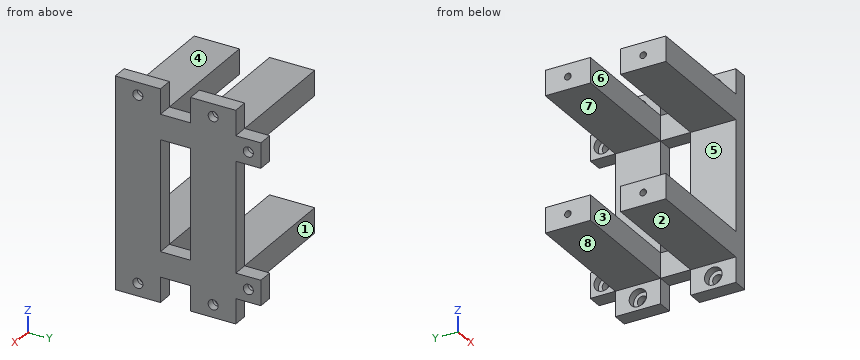
```python
from build123d import *

# Parameters (mm, degrees)
SKETCH_1_W           = 32
SKETCH_1_H           = 24
EXTRUDE_1_DEPTH      = 23.8
SKETCH_7_R           = 0.65
CUT_EXTRUDE_1_DEPTH  = 2
SKETCH_8_OUTSIDE_W   = 43.31
SKETCH_8_OUTSIDE_H   = 35.31
SKETCH_8_OUTSIDE_W_2 = 5
SKETCH_8_OUTSIDE_H_2 = 9
CUT_EXTRUDE_2_DEPTH  = 32.087618114
SKETCH_9_R           = 1
SKETCH_9_W           = 22
SKETCH_9_H           = 6
EXTRUDE_2_DEPTH      = 3
SKETCH_11_R          = 1.75
CUT_EXTRUDE_3_DEPTH  = 1.5


with BuildPart() as part:
    # Sketch 1 → Extrude 1 (new body)
    with BuildSketch(Plane(origin=(0, 0, 0), x_dir=(0, 0, -1), z_dir=(1, 0, 0))):
        Rectangle(SKETCH_1_W, SKETCH_1_H)
    extrude(amount=EXTRUDE_1_DEPTH)

    # Sketch 7 → Cut-Extrude 1 (cut)
    with BuildSketch(Plane.ZY):
        with Locations((13.5, 7.5)):
            Circle(SKETCH_7_R)
        with Locations((13.5, -7.5)):
            Circle(SKETCH_7_R)
        with Locations((-13.5, -7.5)):
            Circle(SKETCH_7_R)
        with Locations((-13.5, 7.5)):
            Circle(SKETCH_7_R)
    extrude(amount=-CUT_EXTRUDE_1_DEPTH, mode=Mode.SUBTRACT)

    # Sketch 8 outside → Cut-Extrude 2 (cut, through all)
    with BuildSketch(Plane.ZY):
        Rectangle(SKETCH_8_OUTSIDE_W, SKETCH_8_OUTSIDE_H)
        with Locations((-13.5, -7.5)):
            Rectangle(SKETCH_8_OUTSIDE_W_2, SKETCH_8_OUTSIDE_H_2, mode=Mode.SUBTRACT)
        with Locations((-13.5, 7.5)):
            Rectangle(SKETCH_8_OUTSIDE_W_2, SKETCH_8_OUTSIDE_H_2, mode=Mode.SUBTRACT)
        with Locations((13.5, -7.5)):
            Rectangle(SKETCH_8_OUTSIDE_W_2, SKETCH_8_OUTSIDE_H_2, mode=Mode.SUBTRACT)
        with Locations((13.5, 7.5)):
            Rectangle(SKETCH_8_OUTSIDE_W_2, SKETCH_8_OUTSIDE_H_2, mode=Mode.SUBTRACT)
    extrude(amount=-CUT_EXTRUDE_2_DEPTH, mode=Mode.SUBTRACT)


with BuildPart() as cut_extrude_2_piece_1:
    # of the separate pieces the step leaves, piece 1, a body of its own (cut_extrude_2_pieces)
    add(part.part.solids().sort_by_distance((0, 12, 16))[0])



with BuildPart() as cut_extrude_2_piece_2:
    # of the separate pieces the step leaves, piece 2, a body of its own (cut_extrude_2_pieces)
    add(part.part.solids().sort_by_distance((0, -12, 16))[0])


with BuildPart() as cut_extrude_2_piece_3:
    # of the separate pieces the step leaves, piece 3, a body of its own (cut_extrude_2_pieces)
    add(part.part.solids().sort_by_distance((0, 3, -11))[0])


with BuildPart() as cut_extrude_2_piece_4:
    # of the separate pieces the step leaves, piece 4, a body of its own (cut_extrude_2_pieces)
    add(part.part.solids().sort_by_distance((0, -12, -11))[0])


with BuildPart() as cut_extrude_2_piece_1_1:
    add(cut_extrude_2_piece_1.part)

    add(cut_extrude_2_piece_2.part)  # Extrude 2 merges Cut-Extrude 2 piece 2

    add(cut_extrude_2_piece_3.part)  # Extrude 2 merges Cut-Extrude 2 piece 3

    add(cut_extrude_2_piece_4.part)  # Extrude 2 merges Cut-Extrude 2 piece 4
    # Sketch 9 → Extrude 2 (add)
    with BuildSketch(Plane(origin=(23.8, 0, 0), x_dir=(0, 0, -1), z_dir=(1, 0, 0))):
        Polygon((16, -3), (16, 3), (21, 3), (21, 12), (16, 12), (16, 17), (11, 17), (11, 12), (-11, 12), (-11, 17), (-16, 17), (-16, 12), (-21, 12), (-21, 3), (-16, 3), (-16, -3), (-21, -3), (-21, -12), (21, -12), (21, -3), align=None)
        with Locations((18.5, 7.5)):
            Circle(SKETCH_9_R, mode=Mode.SUBTRACT)
        with Locations((13.5, 14.5)):
            Circle(SKETCH_9_R, mode=Mode.SUBTRACT)
        with Locations((-18.5, -7.5)):
            Circle(SKETCH_9_R, mode=Mode.SUBTRACT)
        with Locations((18.5, -7.5)):
            Circle(SKETCH_9_R, mode=Mode.SUBTRACT)
        Rectangle(SKETCH_9_W, SKETCH_9_H, mode=Mode.SUBTRACT)
        with Locations((-18.5, 7.5)):
            Circle(SKETCH_9_R, mode=Mode.SUBTRACT)
        with Locations((-13.5, 14.5)):
            Circle(SKETCH_9_R, mode=Mode.SUBTRACT)
    extrude(amount=EXTRUDE_2_DEPTH)

    # Sketch 11 → Cut-Extrude 3 (cut)
    with BuildSketch(Plane.ZY.offset(-23.8)):
        with Locations((-18.5, -7.5)):
            Circle(SKETCH_11_R)
        with Locations((-13.5, -14.5)):
            Circle(SKETCH_11_R)
        with Locations((-18.546966213, 7.5)):
            Circle(SKETCH_11_R)
        with Locations((13.5, -14.5)):
            Circle(SKETCH_11_R)
        with Locations((18.5, -7.5)):
            Circle(SKETCH_11_R)
        with Locations((18.5, 7.5)):
            Circle(SKETCH_11_R)
        with Locations((13.5, 14.5)):
            Circle(SKETCH_11_R)
        with Locations((-13.5, 14.5)):
            Circle(SKETCH_11_R)
    extrude(amount=-CUT_EXTRUDE_3_DEPTH, mode=Mode.SUBTRACT)


solid = cut_extrude_2_piece_1_1.part
```
Could you check a few things on this model? Use its own coordinates, in mm. Face numbers are marked on the shaded views. A direction names the side the tool comes from. Round coordinates to 2 decimals unless told otherwise and drop trailing zeros. Loops run counter-clockwise (first coordinate to the right, second up) from the corner with the lowest first, then second, coordinate; pieces in that order, holes last. Notation, with made-up numbers: (10, 59.25) - (50, 59.25) arc R26 cw to (50, 97.25) - close; hole circle Ø2 at (38.5, -39.5). An arc over 180 degrees is marked (long way). Use CSV: the item, a comma, the result in double quotes.
Item 1: If we section it at A-A on x = 11.75: List the corners of the cut face in (y, z) for me, then the cut area to 3 significant figures.
Here are the results:
outline,"(-12, -16) - (-3, -16) - (-3, -11) - (-12, -11) - close; (-12, 11) - (-3, 11) - (-3, 16) - (-12, 16) - close; (3, -16) - (12, -16) - (12, -11) - (3, -11) - close; (3, 11) - (12, 11) - (12, 16) - (3, 16) - close"
area,"180 mm²"
Item 2: Will these pins go through, and if not, where does the flat tip stop? pin 1 (12 mm diameter, centred on x = 7.5, y = -4, fed in from +Z); pin 2 (0.9 mm diameter, centred on x = 26, y = 14, fed in from -Z); pin 3 (3 mm diameter, centred on y = 7.5, z = 18.5, fed in from -X).
Here are the results:
pin 1,"stops at z = 16"
pin 2,"stops at z = -16"
pin 3,"stops at x = 25.3"
Item 3: If we section it at C-C on z = 13.5: List the corners of the cut face in (x, y) for me, then the cut area to 3 significant figures.
Here are the results:
outline,"(0, -12) - (26.8, -12) - (26.8, 13.5) - (25.3, 13.5) - (25.3, 12.75) - (23.8, 12.75) - (23.8, 12) - (0, 12) - (0, 8.15) - (2, 8.15) - (2, 6.85) - (0, 6.85) - (0, 3) - (23.8, 3) - (23.8, -3) - (0, -3) - (0, -6.85) - (2, -6.85) - (2, -8.15) - (0, -8.15) - close; (23.8, 16.25) - (25.3, 16.25) - (25.3, 15.5) - (26.8, 15.5) - (26.8, 17) - (23.8, 17) - close"
area,"502 mm²"
Item 4: For the marked faces 1, 2, 3 and 4, which set-ups out of +Z, -Z, +X, -X, +Y, -Y let a thin tool reach every point of the face, with its end or its side?
Here are the results:
face 1,"+Z, -Z, -X, +Y"
face 2,"-Z, -X, +Y, -Y"
face 3,"+Z, -Z, -X"
face 4,"+Z, -X, +Y, -Y"
Item 5: I need wall thicknesses on L1, parallel to Z at x = 26.1, y = 7.5; L2, parallel to Y at x = 25.65, z = 18.5; L3, parallel to Y at x = 0.8, z = -13.5. Which ranges of each line are inside material? Lowest first, please. Write a range as [from, to].
Here are the results:
L1,"z = [-21, -19.5], [-17.5, 17.5], [19.5, 21]"
L2,"y = [-12, -8.5], [-6.5, -3], [3, 6.5], [8.5, 12]"
L3,"y = [-12, -8.15], [-6.85, -3], [3, 6.85], [8.15, 12]"
Item 6: If we section it at B-B on y = 14.5: List the corners of the cut face in (x, z) for me, then the cut area to 3 significant figures.
Here are the results:
outline,"(23.8, -16) - (26.8, -16) - (26.8, -14.5) - (25.3, -14.5) - (25.3, -15.25) - (23.8, -15.25) - close; (23.8, -11.75) - (25.3, -11.75) - (25.3, -12.5) - (26.8, -12.5) - (26.8, -11) - (23.8, -11) - close; (23.8, 11) - (26.8, 11) - (26.8, 12.5) - (25.3, 12.5) - (25.3, 11.75) - (23.8, 11.75) - close; (23.8, 15.25) - (25.3, 15.25) - (25.3, 14.5) - (26.8, 14.5) - (26.8, 16) - (23.8, 16) - close"
area,"13.5 mm²"
Item 7: If we section it at D-D on z = 18.5: List the corners of the cut face in (x, y) for me, then the cut area to 3 significant figures.
Here are the results:
outline,"(23.8, -12) - (26.8, -12) - (26.8, -8.5) - (25.3, -8.5) - (25.3, -9.25) - (23.8, -9.25) - close; (23.8, -5.75) - (25.3, -5.75) - (25.3, -6.5) - (26.8, -6.5) - (26.8, -3) - (23.8, -3) - close; (23.8, 3) - (26.8, 3) - (26.8, 6.5) - (25.3, 6.5) - (25.3, 5.75) - (23.8, 5.75) - close; (23.8, 9.25) - (25.3, 9.25) - (25.3, 8.5) - (26.8, 8.5) - (26.8, 12) - (23.8, 12) - close"
area,"37.5 mm²"
Item 8: If we mould it in two halves opening along Z, with no side actions, what happens to the marked faces 5, 6, 7 and 8? For each: pulls with the +Z half, pulls with the -Z half, needs draft (parallel to the pull), parting line crosses it, or undercut.
Here are the results:
face 5,"undercut"
face 6,"needs draft"
face 7,"undercut"
face 8,"pulls with the -Z half"
